Autodesk Inventor part; units mm, degrees
ref_plane "YZ Plane" through (0, 0, 0) normal (1, 0, 0) x (0, 1, 0)
ref_plane "XZ Plane" through (0, 0, 0) normal (0, 1, 0) x (-1, 0, 0)
ref_plane "XY Plane" through (0, 0, 0) normal (0, 0, 1) x (1, 0, 0)
sketch "스케치4" plane through (0, 0, 0) normal (0, 0, 1) x (1, 0, 0)
  circle A0 centre (0, 0) radius 30
  dimension "d28" = 60
extrude "돌출4" add sketch "스케치4" along normal blind 7
sketch "스케치5" plane through (0, 0, 7) normal (0, 0, 1) x (1, 0, 0)
  circle A0 centre (0, 0) radius 16
  dimension "d31" = 32
extrude "돌출5" add sketch "스케치5" along normal blind 4
sketch "스케치6" plane through (0, 0, 0) normal (0, 0, -1) x (-1, 0, 0)
  circle A0 centre (0, 0) radius 17.5
  dimension "d34" = 35
extrude "돌출6" add sketch "스케치6" along normal blind 4
sketch "스케치8" plane through (0, 0, 11) normal (0, 0, 1) x (1, 0, 0)
  circle A0 centre (0, 0) radius 11
  dimension "d41" = 22
extrude "돌출8" cut sketch "스케치8" against normal blind 4
sketch "스케치9" plane through (0, 0, -4) normal (0, 0, -1) x (-1, 0, 0)
  circle A0 centre (0, 0) radius 9.5
  dimension "d44" = 19
extrude "돌출9" cut sketch "스케치9" against normal blind 4
sketch "스케치11" plane through (0, 0, 7) normal (0, 0, 1) x (1, 0, 0)
  circle A0 centre (0, 0) radius 4
  dimension "d49" = 8
extrude "돌출10" cut sketch "스케치11" against normal up to next
sketch "스케치12" plane through (0, 0, 7) normal (0, 0, 1) x (1, 0, 0)
  circle A0 centre (0, 24) radius 3
  point P0 (0, 0)
  dimension "d61" = 6
  dimension "d62" = 24
hole "구멍1" at (0, 24, 7) direction (0, 0, -1) diameter 3.4 end through all counterbore diameter 6 counterbore depth 3.3
pattern_circular "원형 패턴2" count 4 over 360 about axis through (0, 0, 7) along (0, 0, -1) of "구멍1"
fillet "모깎기2" radius 3 4 edges at (-16, 0, 11) (-30, 0, 7) (-16, 0, 7) (9.5, 0, 0)
properties part number "도면2-3번"
Can you work these out from the model? Positions are in its coordinate system, mm. A direction names the side the tool comes from. Round coordinates to 2 decimals unless told otherwise and drop trailing zeros. Order: outer loops, then holes, each group sorted by start corner. A loop starts at its lowest first (then second) coordinate and runs counter-clockwise, first axis right, second up. Notation, with made-up numbers: M -33.75,41.5 L -2.75,41.5 A9 ccw -2.75,57.5 Z; hole C -30.75,-14.75 d6. An arc over 180 degrees is marked long. Use a Markdown table: item, result.
1) If I drill on line 1 along Y through (x, z) = (0, -3.5); line 2 along X through (y, z) = (-1.5, 1); line 3 along Z through (x, y) = (-11, -19), over which ranges is the centre line in solid material (lowest first)?
Geometry says:
| item | result |
|---|---|
| line 1 | y = -17.5 to -9.5, 9.5 to 17.5 |
| line 2 | x = -29.96 to -24.8, -23.2 to -3.71, 3.71 to 23.2, 24.8 to 29.96 |
| line 3 | z = 0 to 7 |
2) I'm going to push flat-ended pins straight in: P1, Ø1.8, axis at x = -1, y = -23, coming from the +Z side; P2, Ø8, axis at x = -24, y = 0, coming from the -Z side; P3, Ø6.5, axis at x = 0, y = 0, coming from the +Z side (1 decimal); P4, Ø1.5, axis at y = 11.5, z = 4.5, coming from the +X side. Where does each tip first touch, or does it pass through?
Geometry says:
| item | result |
|---|---|
| P1 | stops at z = 3.7 |
| P2 | stops at z = 0 |
| P3 | passes through |
| P4 | stops at x = 27.98 |
3) If we mould it in two halves opening along Y, with no side actions, what happens to faces 1 (the face through (-29.97, -1.32, 1.97)), 2 (the face through (13, -13, 0)), 3 (the face through (-24, 2, 3.7))? For each: +Y half, -Y half, draft (parallel to the pull), parting line (faces both ways), or undercut.
Geometry says:
| item | result |
|---|---|
| face 1 | parting line |
| face 2 | draft |
| face 3 | undercut |
4) On a 3-axis mill with a long thin cutter (end or side, diameter ignored), from which of +Z, -Z, +X, -X, +Y, -Y can I reach the whole of each face in a straight line? I mean faces 4 (the face through (22.43, -0.65, 1.82)), 5 (the face through (2, 24, 3.7)), 6 (the face through (13.887, 10.648, -1.972)). Say none if no direction works.
Geometry says:
| item | result |
|---|---|
| face 4 | +Z, -Z |
| face 5 | +Z |
| face 6 | -Z |
5) Imagine slicing it at C-C (z = -0.75). List the corners of the cut face in (x, y) for me, then the cut area to 3 significant figures.
Geometry says:
| item | result |
|---|---|
| outline | C 0,0 d35; hole C 0,0 d16.97 |
| area | 736 mm² |
6) Imagine slicing it at A-A (x = 0). Give the number of separate pieces and of enclosed holes in the cut face, then the cut area to 3 significant figures.
Geometry says:
| item | result |
|---|---|
| separate pieces | 4 |
| enclosed holes | 0 |
| area | 402 mm² |
